Verification items for this drawing (mm, ordinates from the low corner). Round coordinates to 2 decimals unless told otherwise and drop trailing zeros. Write each loop counter-clockwise with the first axis right and the second up, starting at its lowest first coordinate (ties: lowest second). Pieces come first, ordered by that corner, then holes. Notation, with made-up numbers: (28, 86) -> (61, 86) arc R25 ccw to (61, 107) -> close; hole circle Ø4 at (67.25, 41). An arc over 180 degrees is marked (long way). One line per question, with ' | ' between items.
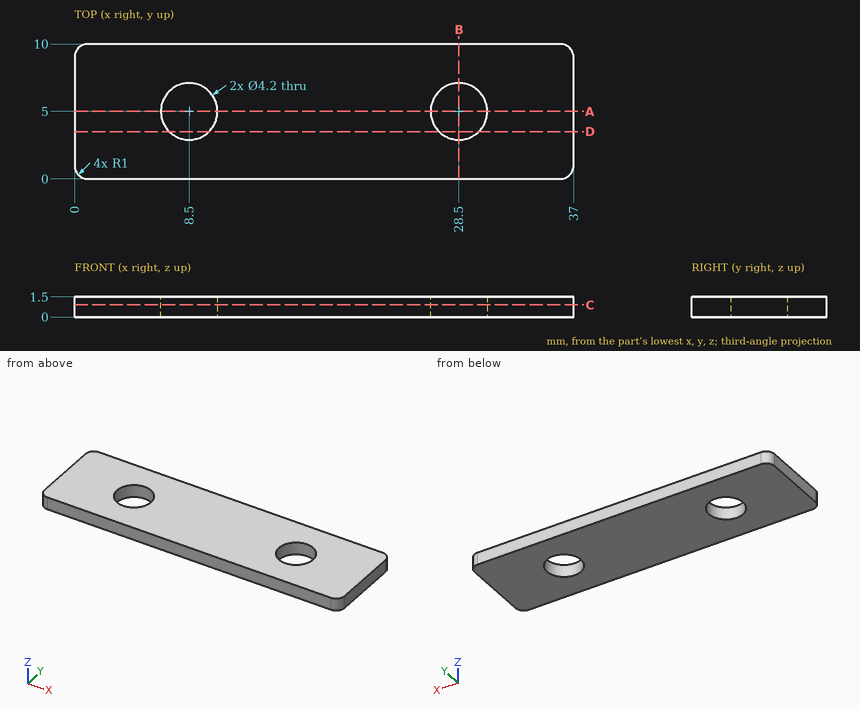
(1) Sectioned sample at B-B on x = 28.5. Record the cut outline in (y, z).
Resolved:
outline: (0, 0) -> (2.9, 0) -> (2.9, 1.5) -> (0, 1.5) -> close; (7.1, 0) -> (10, 0) -> (10, 1.5) -> (7.1, 1.5) -> close
(2) Sectioned sample at A-A on y = 5. Record the cut outline in (x, z).
Resolved:
outline: (0, 0) -> (6.4, 0) -> (6.4, 1.5) -> (0, 1.5) -> close; (10.6, 0) -> (26.4, 0) -> (26.4, 1.5) -> (10.6, 1.5) -> close; (30.6, 0) -> (37, 0) -> (37, 1.5) -> (30.6, 1.5) -> close
(3) Go/stop test with a flat-tipped pin: pin 1 (5 mm diameter, centred on x = 8.5, y = 5, fed in from -Z). Record where the tip stops, or that it passes through.
Resolved:
pin 1: stops at z = 0
(4) Sectioned sample at D-D on y = 3.5. Record the cut outline in (x, z), then the cut area to 3 significant figures.
Resolved:
outline: (0, 0) -> (7.03, 0) -> (7.03, 1.5) -> (0, 1.5) -> close; (9.97, 0) -> (27.03, 0) -> (27.03, 1.5) -> (9.97, 1.5) -> close; (29.97, 0) -> (37, 0) -> (37, 1.5) -> (29.97, 1.5) -> close | area: 46.7 mm2
(5) Material ranges on line 1 (X direction, y = 5, z = 0.65); line 2 (Y direction, x = 28.5, z = 0.65); line 3 (X direction, y = 3.75, z = 0.45), recorded low to high.
Resolved:
line 1: x = 0 to 6.4, 10.6 to 26.4, 30.6 to 37 | line 2: y = 0 to 2.9, 7.1 to 10 | line 3: x = 0 to 6.81, 10.19 to 26.81, 30.19 to 37
(6) Sectioned sample at C-C on z = 0.9. Record the cut outline in (x, y).
Resolved:
outline: (0, 1) arc R1 ccw to (1, 0) -> (36, 0) arc R1 ccw to (37, 1) -> (37, 9) arc R1 ccw to (36, 10) -> (1, 10) arc R1 ccw to (0, 9) -> close; hole circle Ø4.2 at (8.5, 5); hole circle Ø4.2 at (28.5, 5)
